Source: three-view drawing plus pictorial views. Frame: mm from the lowest corner of the part. A direction names the side the tool comes from. Coordinates: 2 decimals unless noted, no trailing zeros. Order: outer loops, then holes, each group sorted by start corner. A loop starts at its lowest first (then second) coordinate and runs counter-clockwise, first axis right, second up. Notation, with made-up numbers: (19, 34.25) -> (77, 34.25) arc R15 cw to (77, 48.25) -> close; hole circle Ø11 at (14.25, 7). An arc over 180 degrees is marked (long way). Use one line per item in the form item = value. Start each with the question number.
1) Ray query, line 1 along Y through (x, z) = (7.5, 35); line 2 along Y through (x, z) = (24, 24.5); line 3 along X through (y, z) = (46, 21). Return the intervals inside material, ascending.
2) Section query B-B on z = 21. Output: boundary loops of the cut face in (x, y), then the cut area to 3 significant figures.
3) Access query for the marked faces 1 and 2. Directions: +Z, -Z, +X, -X, +Y, -Y. A direction counts if a zero-diameter tool reaches every point of the face in a straight line with its end or side. Return the directions, or none.
4) Section query D-D on z = 15.5. Output: boundary loops of the cut face in (x, y), then the cut area to 3 significant figures.
5) Section query A-A on x = 21. Output: boundary loops of the cut face in (y, z), then the cut area to 3 significant figures.
6) Section query C-C on y = 38. Output: boundary loops of the cut face in (x, z).
7) Pin query (flat end, axial travel): pin 1 (2.5 mm diameter, centred on x = 21, y = 38.5, fed in from -Z); pin 2 (3 mm diameter, centred on x = 36.495, z = 5.505, fed in from +Y); pin 3 (0.6 mm diameter, centred on x = 36.5, z = 6, fed in from +Y). Return the tip coordinate at first contact, or that it passes through.
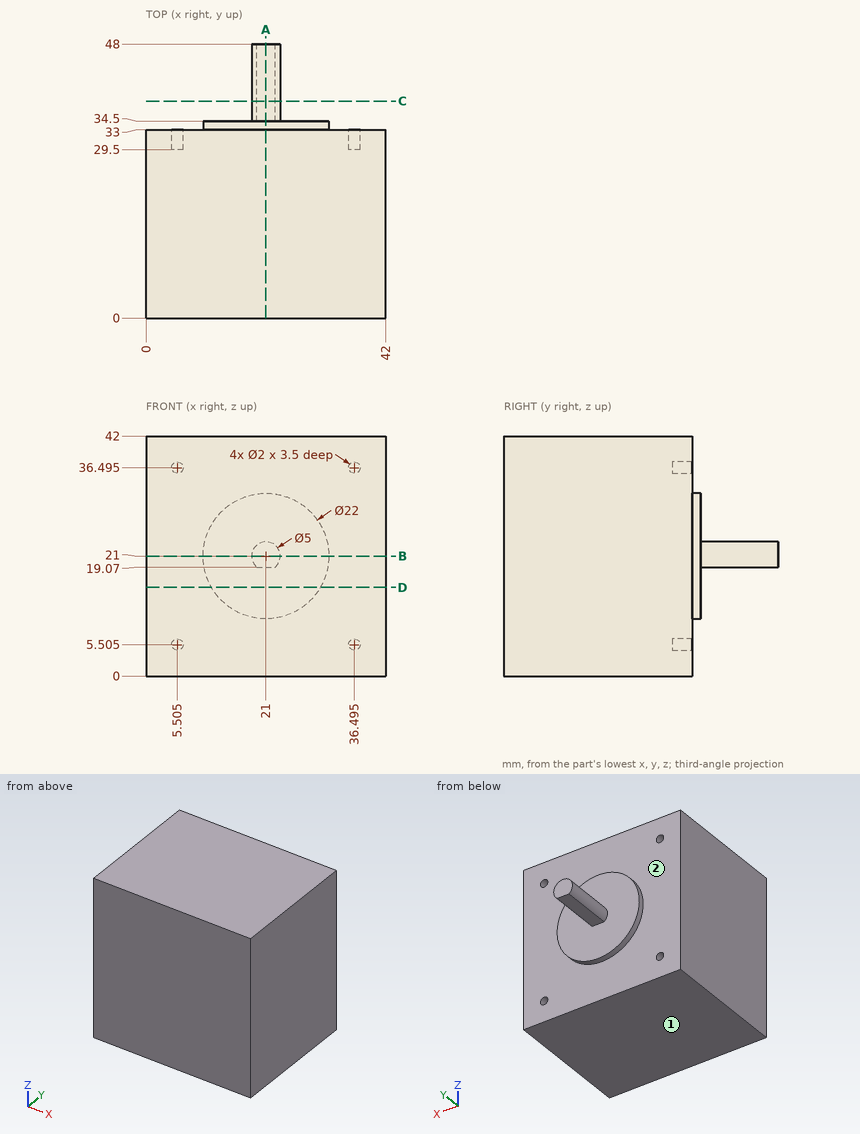
Answers below:
q1.line_1 = 0 to 33
q1.line_2 = 0 to 34.5
q1.line_3 = 18.5 to 23.5
q2.outline = (0, 0) -> (42, 0) -> (42, 33) -> (32, 33) -> (32, 34.5) -> (23.5, 34.5) -> (23.5, 48) -> (18.5, 48) -> (18.5, 34.5) -> (10, 34.5) -> (10, 33) -> (0, 33) -> close
q2.area = 1,490 mm^2
q3.face_1 = -Z, +X, -X, +Y, -Y
q3.face_2 = +Y
q4.outline = (0, 0) -> (42, 0) -> (42, 33) -> (30.53, 33) -> (30.53, 34.5) -> (11.47, 34.5) -> (11.47, 33) -> (0, 33) -> close
q4.area = 1,410 mm^2
q5.outline = (0, 0) -> (33, 0) -> (33, 10) -> (34.5, 10) -> (34.5, 19.07) -> (48, 19.07) -> (48, 23.5) -> (34.5, 23.5) -> (34.5, 32) -> (33, 32) -> (33, 42) -> (0, 42) -> close
q5.area = 1,480 mm^2
q6.outline = (19.41, 19.07) -> (22.59, 19.07) arc R2.5 ccw (long way) to start
q7.pin_1 = 19.07
q7.pin_2 = 33
q7.pin_3 = 29.5
